Source: CAD feature listing. Evaluate the final solid. Frame: model axes, mm. A direction names the side the tool comes from. Give positions to 0.01 mm unless a question says otherwise; leave off trailing zeros. Write each loop counter-clockwise with the first axis right and the second up, starting at its lowest first coordinate (ties: lowest second). Pieces come first, ordered by that corner, then holes. Notation, with made-up numbers: M -34.5,34 L 5.5,34 A32 cw 5.5,73 Z; hole C -28.5,-19 d11. An arc over 180 degrees is marked long. Return JSON: item names as keys, results as strings.
```python
from build123d import *

# Parameters (mm, degrees)
EXTRUDE_1_DEPTH     = 2.4
SKETCH_2_R          = 1.25
CUT_EXTRUDE_1_DEPTH = 41.333112947
CUT_EXTRUDE_START   = -1.5
SKETCH_2_3_R        = 2
SKETCH_2_3_R_2      = 1.25
CUT_EXTRUDE_2_DEPTH = 0.9
SKETCH_3_R          = 2.55
CUT_EXTRUDE_3_DEPTH = 41.333112947
SKETCH_4_R          = 1.5
EXTRUDE_2_DEPTH     = 2.5


with BuildPart() as part:
    # 草图1 → 凸台-拉伸1 (new body)
    with BuildSketch(Plane.XY):
        with BuildLine():
            Line((0, -10), (39, -10))
            Line((39, -10), (39, 10))
            Line((39, 10), (0, 10))
            ThreePointArc((0, 10), (-10, 0), (0, -10))
        make_face()
    extrude(amount=EXTRUDE_1_DEPTH)

    # 草图2 → 切除-拉伸1 (cut, through all)
    with BuildSketch(Plane(origin=(0, 0, 0), x_dir=(-1, 0, 0), z_dir=(0, 0, -1))):
        with Locations((-33, 6)):
            Circle(SKETCH_2_R)
        with Locations((-33, -6)):
            Circle(SKETCH_2_R)
        with Locations((-26, 0)):
            Circle(SKETCH_2_R)
    extrude(amount=-CUT_EXTRUDE_1_DEPTH, mode=Mode.SUBTRACT)

    # 草图2<3> → 切除-拉伸2 (cut)
    # profile 1 of 3: a face of its own
    with BuildSketch(Plane(origin=(0, 0, 0), x_dir=(-1, 0, 0), z_dir=(0, 0, -1)).offset(CUT_EXTRUDE_START)):
        with Locations(Location((-33, 6, 0), (0, 0, 180))):
            Circle(SKETCH_2_3_R)
        with Locations((-33, 6)):
            Circle(SKETCH_2_3_R_2, mode=Mode.SUBTRACT)
    # profile 2 of 3: a face of its own
    with BuildSketch(Plane(origin=(0, 0, 0), x_dir=(-1, 0, 0), z_dir=(0, 0, -1)).offset(CUT_EXTRUDE_START)):
        with Locations(Location((-33, -6, 0), (0, 0, 180))):
            Circle(SKETCH_2_3_R)
        with Locations((-33, -6)):
            Circle(SKETCH_2_3_R_2, mode=Mode.SUBTRACT)
    # profile 3 of 3: a face of its own
    with BuildSketch(Plane(origin=(0, 0, 0), x_dir=(-1, 0, 0), z_dir=(0, 0, -1)).offset(CUT_EXTRUDE_START)):
        with Locations(Location((-26, 0, 0), (0, 0, 180))):
            Circle(SKETCH_2_3_R)
        with Locations((-26, 0)):
            Circle(SKETCH_2_3_R_2, mode=Mode.SUBTRACT)
    extrude(amount=-CUT_EXTRUDE_2_DEPTH, mode=Mode.SUBTRACT)

    # 草图3 → 切除-拉伸3 (cut, through all)
    with BuildSketch(Plane.XY.offset(2.4)):
        Circle(SKETCH_3_R)
    extrude(amount=-CUT_EXTRUDE_3_DEPTH, mode=Mode.SUBTRACT)

    # 草图4 → 凸台-拉伸2 (add)
    with BuildSketch(Plane.XY.offset(2.4)):
        with Locations((11.8, -4)):
            Circle(SKETCH_4_R)
        with Locations((11.8, 4)):
            Circle(SKETCH_4_R)
    extrude(amount=EXTRUDE_2_DEPTH)


solid = part.part
```
1) Cut plane A-A, the plane z = 0.55. Return the cut outline in (x, y).
Numbers:
{"outline": "M 0,-10 L 39,-10 L 39,10 L 0,10 A10 ccw Z; hole C 0,0 d5.1; hole C 26,0 d2.5; hole C 33,-6 d2.5; hole C 33,6 d2.5"}
2) Cut plane C-C, the plane x = 26.5. Return the cut outline in (y, z).
Numbers:
{"outline": "M -10,0 L -1.15,0 L -1.15,1.5 L -1.94,1.5 L -1.94,2.4 L -10,2.4 Z; M 1.15,0 L 10,0 L 10,2.4 L 1.94,2.4 L 1.94,1.5 L 1.15,1.5 Z"}
3) Cut plane D-D, the plane z = 4.45. Return the cut outline in (x, y).
Numbers:
{"outline": "C 11.8,-4 d3; C 11.8,4 d3"}
4) Contact query for flat-ended pins moving along their axis: pin 1 Ø5 at (x, y) = (33, 6) entering from +Z; pin 2 Ø1.2 at (x, y) = (33.5, 6.5) entering from +Z. Output: stop coordinate, or through.
Numbers:
{"pin 1": "stops at z = 2.4", "pin 2": "stops at z = 1.5"}
5) Line query: line 1 (Y direction, x = 33, z = 0.65); line 2 (Y direction, x = 33, z = 1.8); line 3 (X direction, y = -0.5, z = 0.9). Output: solid intervals per line, ascending. Write a range as [from, to].
Numbers:
{"line 1": "y = [-10, -7.25], [-4.75, 4.75], [7.25, 10]", "line 2": "y = [-10, -8], [-4, 4], [8, 10]", "line 3": "x = [-9.99, -2.5], [2.5, 24.85], [27.15, 39]"}
6) Set-up query: faces 5 (the face through (20, 10, 1)), 6 (the face through (34.908, -6.601, 1.944)). Return all of +Z, -Z, +X, -X, +Y, -Y with unobstructed straight access to the full face (end or side cutting, diameter ignored); none if empty.
Numbers:
{"face 5": "+Z, -Z, +X, -X, +Y", "face 6": "+Z"}
7) Draft query along X for faces 1 (the face through (27, -1, 1.5)), 2 (the face through (14, 0, 0)), 3 (the face through (32, -5, 1.5)), 4 (the face through (13.23, -3.55, 3.63)). Return one class per face: released by +X, released by -X, zero draft, split by the parting line, or undercut.
Numbers:
{"face 1": "undercut", "face 2": "zero draft", "face 3": "undercut", "face 4": "split by the parting line"}
8) Cut plane B-B, the plane x = 33. Return the cut outline in (y, z), then the cut area to 3 significant figures.
Numbers:
{"outline": "M -10,0 L -7.25,0 L -7.25,1.5 L -8,1.5 L -8,2.4 L -10,2.4 Z; M -4.75,0 L 4.75,0 L 4.75,1.5 L 4,1.5 L 4,2.4 L -4,2.4 L -4,1.5 L -4.75,1.5 Z; M 7.25,0 L 10,0 L 10,2.4 L 8,2.4 L 8,1.5 L 7.25,1.5 Z", "area": "33.3 mm²"}
